Build history of the part. All positions in model axes, mm. Give positions to 0.01 mm unless a question says otherwise; leave off trailing zeros. Loops run counter-clockwise (first coordinate to the right, second up) from the corner with the lowest first, then second, coordinate; pieces in that order, holes last.
1) Flat gauge pins, fed straight in: P1, Ø1, axis at y = 83.5, z = 0.5, coming from the -X side; P2, Ø3, axis at x = 25.4, y = -195.58, coming from the +Z side; P3, Ø3, axis at y = 82, z = -1.5, coming from the -X side. Where does each tip first touch, or does it go through?
2) Band-saw the part on B-B on x = 230.5. List the corners of the cut face in (y, z).
3) Band-saw the part on C-C on y = 85.5. List the corners of the cut face in (x, z).
4) Wall check: line 1 (X direction, y = -246.38, z = -0.1); line 2 (Y direction, x = 25.4, z = -1.4); line 3 (X direction, y = -144.78, z = 0.9). Give the ranges that are in metal, low to high.
5) Band-saw the part on A-A on z = -0.5. State how many separate pieces and enclosed holes the cut face has, then the cut area to 3 significant figures.
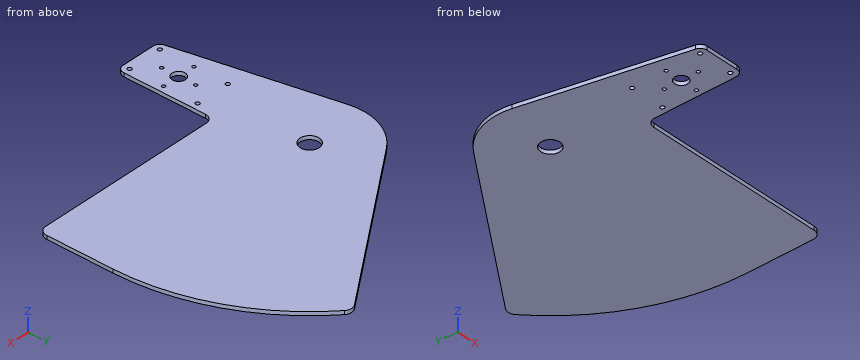
```python
from build123d import *

# Parameters (mm, degrees)
SKETCH1_R               = 86.36
SKETCH1_R_2             = 14.2875
BOSS_EXTRUDE1_DEPTH     = 2.75
SKETCH2_R               = 33.4
SKETCH2_R_2             = 9.906
SKETCH2_R_3             = 2.5
BOSS_EXTRUDE2_DEPTH     = 5.5
FILLET2_R               = 12.7
SKETCH4_R               = 3
BOSS_EXTRUDE3_DEPTH     = 5.5
CUT_EXTRUDE1_DEPTH      = 419.082521041
CUT_EXTRUDE1_DEPTH_BACK = 419.082521041
SKETCH4_3_R             = 3
FILLET3_R               = 12.7


with BuildPart() as part:
    # Sketch1 → Boss-Extrude1 (new, symmetric)
    # profile 1 of 3: a face of its own
    with BuildSketch(Plane.XY):
        Circle(SKETCH1_R)
        Circle(SKETCH1_R_2, mode=Mode.SUBTRACT)
    # profile 2 of 3: a face of its own
    with BuildSketch(Plane.XY):
        with BuildLine():
            Line((0, -86.36), (0, -111.76))
            Line((0, -111.76), (310.711670846, -111.76))
            ThreePointArc((310.711670846, -111.76), (325.291433728, -56.723215206), (330.2, 0))
            ThreePointArc((330.2, 0), (299.066021409, 139.96983546), (211.535222055, 253.544650565))
            Line((211.535222055, 253.544650565), (-49.534061043, 70.741970545))
            ThreePointArc((-49.534061043, 70.741970545), (39.876610239, 76.602255553), (86.36, 0))
            ThreePointArc((86.36, 0), (61.065741623, -61.065741623), (0, -86.36))
        make_face()
    # profile 3 of 3: a face of its own
    with BuildSketch(Plane.XY):
        with BuildLine():
            ThreePointArc((330.2, 0), (325.291433728, -56.723215206), (310.711670846, -111.76))
            Line((310.711670846, -111.76), (330.2, -111.76))
            Line((330.2, -111.76), (330.2, 0))
        make_face()
    extrude(amount=BOSS_EXTRUDE1_DEPTH, both=True)

    # Sketch2 → Boss-Extrude2 (add)
    # profile 1 of 2: a face of its own
    with BuildSketch(Plane.XY.offset(2.75)):
        with BuildLine():
            ThreePointArc((-32.152177301, -204.624196748), (-4.564935824, -162.493426274), (33.4, -195.58))
            Line((33.4, -195.58), (33.4, -111.76))
            Line((33.4, -111.76), (0, -111.76))
            Line((0, -111.76), (0, -86.36))
            ThreePointArc((0, -86.36), (-52.146556012, -68.838842931), (-83.133593763, -23.384935065))
            Line((-83.133593763, -23.384935065), (-32.152177301, -204.624196748))
        make_face()
    # profile 2 of 2: a face of its own
    with BuildSketch(Plane.XY.offset(2.75)):
        with Locations((0, -195.58)):
            Circle(SKETCH2_R)
        with Locations((0, -195.58)):
            Circle(SKETCH2_R_2, mode=Mode.SUBTRACT)
        with Locations((0, -170.18)):
            Circle(SKETCH2_R_3, mode=Mode.SUBTRACT)
        with Locations((25.4, -195.58)):
            Circle(SKETCH2_R_3, mode=Mode.SUBTRACT)
        with Locations((0, -220.98)):
            Circle(SKETCH2_R_3, mode=Mode.SUBTRACT)
        with Locations((-25.4, -195.58)):
            Circle(SKETCH2_R_3, mode=Mode.SUBTRACT)
    extrude(amount=-BOSS_EXTRUDE2_DEPTH)

    # Fillet2
    fillet2_edges = [part.edges().sort_by_distance(p)[0] for p in [
        (211.535222055, 253.544650565, 0),
        (330.2, -111.76, 0),
        (33.4, -111.76, 0),
    ]]
    fillet(fillet2_edges, radius=FILLET2_R)

    # Sketch4 → Boss-Extrude3 (add)
    with BuildSketch(Plane.XY.offset(2.75)):
        with BuildLine():
            ThreePointArc((-83.133593763, -23.384935065), (-83.834442875, -20.732481468), (-84.450685864, -18.05910455))
            Line((-84.450685864, -18.05910455), (-35.178912212, -248.471142259))
            ThreePointArc((-35.178912212, -248.471142259), (-31.688424978, -254.155327086), (-25.4, -256.38))
            Line((-25.4, -256.38), (25.4, -256.38))
            ThreePointArc((25.4, -256.38), (32.743767081, -253.16742109), (35.369047914, -245.593817011))
            Line((35.369047914, -245.593817011), (35.369047914, -117.66760224))
            ThreePointArc((35.369047914, -117.66760224), (33.902190945, -120.923977623), (33.4, -124.46))
            Line((33.4, -124.46), (33.4, -195.58))
            ThreePointArc((33.4, -195.58), (4.564935824, -228.666573726), (-32.152177301, -204.624196748))
            Line((-32.152177301, -204.624196748), (-83.133593763, -23.384935065))
        make_face()
        with Locations((-25.4, -246.38)):
            Circle(SKETCH4_R, mode=Mode.SUBTRACT)
        with Locations((25.4, -246.38)):
            Circle(SKETCH4_R, mode=Mode.SUBTRACT)
    extrude(amount=-BOSS_EXTRUDE3_DEPTH)

    # Sketch4<3> → Cut-Extrude1 (cut, two sides: drawn at the far end of the back side and taken through both)
    with BuildSketch(Plane.XY.offset(2.75).offset(-CUT_EXTRUDE1_DEPTH_BACK)):
        with Locations((-25.4, -144.78)):
            Circle(SKETCH4_3_R)
        with Locations((25.4, -144.78)):
            Circle(SKETCH4_3_R)
    extrude(amount=CUT_EXTRUDE1_DEPTH + CUT_EXTRUDE1_DEPTH_BACK, mode=Mode.SUBTRACT)

    # Fillet3
    # the kernel refuses this fillet: 12.7 mm, written as the material it adds along each edge
    with BuildSketch(Plane(origin=(35.369047914, -117.66760224, 2.75), x_dir=(0.9067040347764744, 0.4217674635626387, 0), z_dir=(0, 0, -1))) as fillet3_piece_1:
        with BuildLine():
            CenterArc((8.650328867, 11.515141242), FILLET3_R, 204.946225236, 90)
            Line((-2.864812375, 6.158694454), (-4.016326499, 5.623049776))
            Line((-4.016326499, 5.623049776), (-1.151514124, -0.535644679))
            Line((-1.151514124, -0.535644679), (-0.686498518, -1.06846609))
            ThreePointArc((-0.686498518, -1.06846609), (12.757076645, -1.981994468), (14.542420333, -1.151514124))
            Line((14.542420333, -1.151514124), (14.006775654, 0))
        make_face()
    extrude(amount=5.5)


solid = part.part
```
Findings below:
1. P1: stops at x = -32.03
1. P2: passes through
1. P3: stops at x = -35.6
2. outline: (-111.76, -2.75) - (236.44, -2.75) - (236.44, 2.75) - (-111.76, 2.75) - close
3. outline: (-28.46, -2.75) - (318.94, -2.75) - (318.94, 2.75) - (-28.46, 2.75) - close
4. line 1: x = -35.63 to -28.4, -22.4 to 22.4, 28.4 to 35.4
4. line 2: y = -256.38 to -249.38, -243.38 to -198.08, -193.08 to -147.78, -141.78 to 123.21
4. line 3: x = -57.35 to -28.4, -22.4 to 22.4, 28.4 to 35.37
5. separate pieces: 1
5. enclosed holes: 10
5. area: 121,000 mm2
